```python
from build123d import *

# Parameters (mm, degrees)
F0_W      = 76.2
F0_H      = 44.45
F1_DEPTH  = 25.4
F2_W      = 25.4
F2_H      = 31.75
F3_DEPTH  = 25.4
F4_R      = 6.5486317255
F5_DEPTH  = 25.4
F6_R      = 6.35
F7_DEPTH  = 25.4
F9_DEPTH  = 25.4
F10_R     = 6.35
F11_DEPTH = 25.4


with BuildPart() as f1:
    # F0 (on Front) → F1 (new body)
    with BuildSketch(Plane.XZ):
        with Locations((38.1, 22.225)):
            Rectangle(F0_W, F0_H)
    extrude(amount=F1_DEPTH)

    # F2 (on face) → F3 (cut)
    with BuildSketch(Plane.XZ.offset(25.4)):
        with Locations((63.5, 28.575)):
            Rectangle(F2_W, F2_H)
        with Locations((12.7, 28.575)):
            Rectangle(F2_W, F2_H)
    extrude(amount=-F3_DEPTH, mode=Mode.SUBTRACT)

    # F4 (on face) → F5 (cut)
    with BuildSketch(Plane.YZ.offset(50.8)):
        with Locations((-12.8986317255, 31.7515534242)):
            Circle(F4_R)
        with BuildLine():
            ThreePointArc((-25.4, 31.75), (-21.6802561211, 40.7302561211), (-12.7, 44.45))
            Line((-12.7, 44.45), (-25.4, 44.45))
            Line((-25.4, 44.45), (-25.4, 31.75))
        make_face()
        with BuildLine():
            ThreePointArc((-12.7, 44.45), (-3.7197438789, 40.7302561211), (0, 31.75))
            Line((0, 31.75), (0, 44.45))
            Line((0, 44.45), (-12.7, 44.45))
        make_face()
    extrude(amount=-F5_DEPTH, mode=Mode.SUBTRACT)

    # F6 (on face) → F7 (cut)
    with BuildSketch(Plane.XY.offset(12.7)):
        with Locations((63.5, -12.7)):
            Circle(F6_R)
    extrude(amount=-F7_DEPTH, mode=Mode.SUBTRACT)

    # F8 (on face) → F9 (cut)
    with BuildSketch(Plane.XY.offset(12.7)):
        with BuildLine():
            ThreePointArc((63.5, 0), (72.4802561211, -3.7197438789), (76.2, -12.7))
            Line((76.2, -12.7), (76.2, 0))
            Line((76.2, 0), (63.5, 0))
        make_face()
        with BuildLine():
            ThreePointArc((76.2, -12.7), (72.4802561211, -21.6802561211), (63.5, -25.4))
            Line((63.5, -25.4), (76.2, -25.4))
            Line((76.2, -25.4), (76.2, -12.7))
        make_face()
    extrude(amount=-F9_DEPTH, mode=Mode.SUBTRACT)

    # F10 (on face) → F11 (cut)
    with BuildSketch(Plane.XY.offset(12.7)):
        with BuildLine():
            ThreePointArc((4.2558507994, -25.4), (0.4710381636, -12.1911505721), (6.809362676, 0))
            Line((6.809362676, 0), (0, 0))
            Line((0, 0), (0, -25.4))
            Line((0, -25.4), (4.2558507994, -25.4))
        make_face()
        with Locations((12.7, -12.7)):
            Circle(F10_R)
    extrude(amount=-F11_DEPTH, mode=Mode.SUBTRACT)


solid = f1.part
```
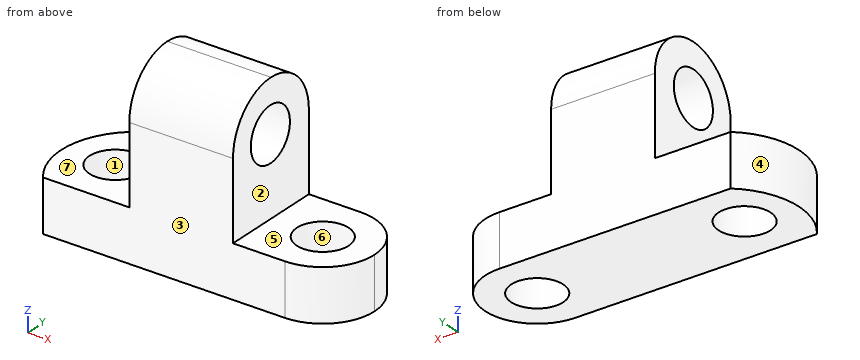
CAD build for the part. Positions are in the model's coordinates, mm. Face numbers are marked on the shaded views. A direction names the side the tool comes from. Round coordinates to 2 decimals unless told otherwise and drop trailing zeros. Loops run counter-clockwise (first coordinate to the right, second up) from the corner with the lowest first, then second, coordinate; pieces in that order, holes last. Notation, with made-up numbers: M 40,57 L 69,57 A20 ccw 69,76 Z; hole C 29.5,64 d3. An arc over 180 degrees is marked long. Use a Markdown table: item, result. Add a question column.
(1) Drill centre lines: line 1 (X direction, y = -14.25, z = 12); line 2 (X direction, y = -18, z = 5.5); line 3 (Z direction, x = 21, y = -13). Where is each one in solid material? Low to high.
(2) Cut at B-B (z = 5.5). Give the cut face in (x, y).
(3) Which spindle directions (+Z, -Z, +X, -X, +Y, -Y) get a long thin tool onto all of the face, cutting with end or side? Do the marked faces 5, 6 and 7. Say none if no direction does.
(4) Pull direction Y, two halves, no side cores. Call the marked faces 1, 2, 3 and 4: +Y half, -Y half, draft (parallel to the pull), parting line (faces both ways), or undercut.
(5) Cut at A-A (x = 12.7). Give the cut face in (y, z), and give its area (3 significant figures).
(6) Cut at C-C (y = -9). Give the cut face in (x, z).
(7) Flat gauge pins, fed straight in: pin 1 (10 mm diameter, centred on y = -3.5, z = 30.5, fed in from +X); pin 2 (1.5 mm diameter, centred on y = -9, z = 32, fed in from +X); pin 3 (6 mm diameter, centred on x = 32, y = -22.5, fed in from +Z); pin 4 (7.5 mm diameter, centred on y = -8.5, z = 21, fed in from -X). Where does each tip first touch, or does it go through?
(8) Cut at D-D (y = -2.75). Give the cut face in (x, z), and give its area (3 significant figures).
Geometry says:
| question | item | result |
|---|---|---|
| 1 | line 1 | x = 0.38 to 6.54, 18.86 to 57.34, 69.66 to 76.11 |
| 1 | line 2 | x = 0.8 to 9.2, 16.2 to 60, 67 to 75.04 |
| 1 | line 3 | z = 0 to 12.7 |
| 2 | outline | M 4.26,-25.4 L 63.5,-25.4 A12.7 ccw 63.5,0 L 6.81,0 A18.56 ccw Z; hole C 12.7,-12.7 d12.7; hole C 63.5,-12.7 d12.7 |
| 3 | face 5 | +Z, +X, +Y, -Y |
| 3 | face 6 | +Z, -Z |
| 3 | face 7 | +Z, -X, +Y, -Y |
| 4 | face 1 | undercut |
| 4 | face 2 | draft |
| 4 | face 3 | -Y half |
| 4 | face 4 | parting line |
| 5 | outline | M -25.4,0 L -19.05,0 L -19.05,12.7 L -25.4,12.7 Z; M -6.35,0 L 0,0 L 0,12.7 L -6.35,12.7 Z |
| 5 | area | 161 mm² |
| 6 | outline | M 1.08,0 L 7.54,0 L 7.54,12.7 L 1.08,12.7 Z; M 17.86,0 L 58.34,0 L 58.34,12.7 L 50.8,12.7 L 50.8,26.49 L 25.4,26.49 L 25.4,12.7 L 17.86,12.7 Z; M 25.4,37.01 L 50.8,37.01 L 50.8,43.9 L 25.4,43.9 Z; M 68.66,0 L 75.65,0 L 75.65,12.7 L 68.66,12.7 Z |
| 7 | pin 1 | stops at x = 50.8 |
| 7 | pin 2 | passes through |
| 7 | pin 3 | stops at z = 42.48 |
| 7 | pin 4 | stops at x = 25.4 |
| 8 | outline | M 4.21,0 L 71.39,0 L 71.39,12.7 L 50.8,12.7 L 50.8,39.64 L 25.4,39.64 L 25.4,12.7 L 4.21,12.7 Z |
| 8 | area | 1,540 mm² |
